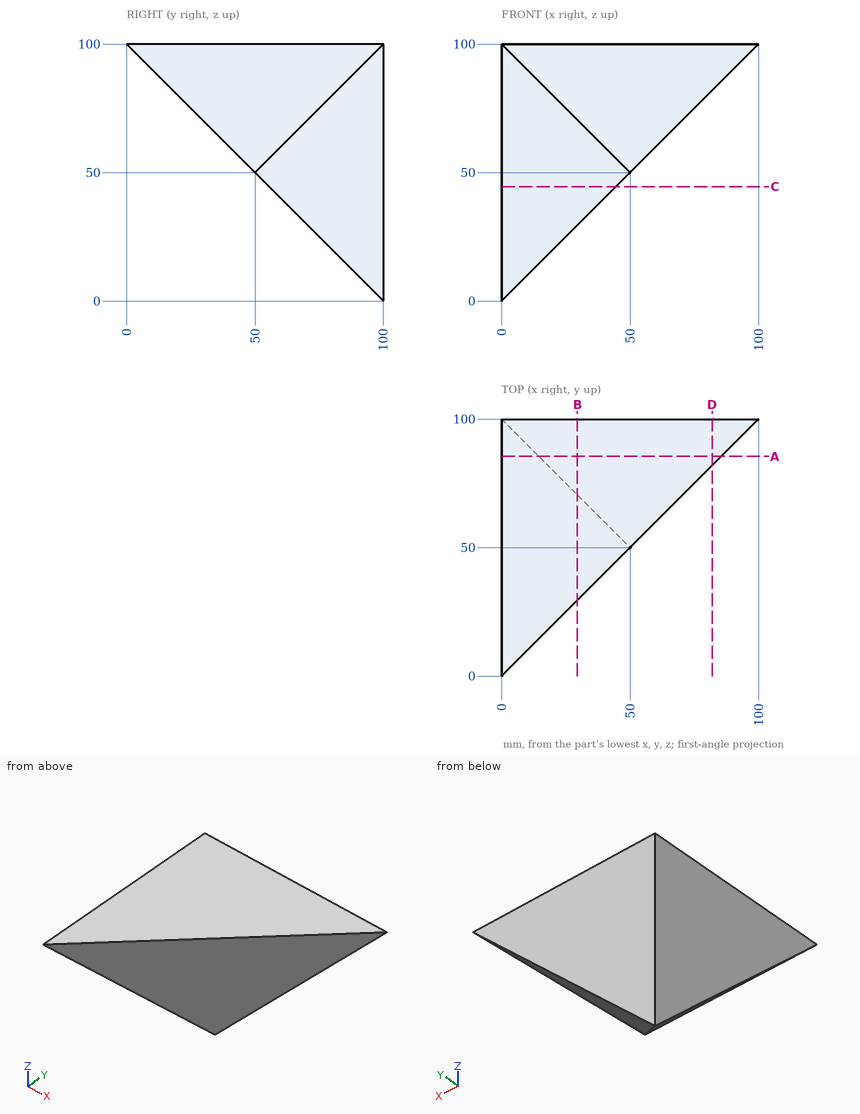
The figure shows three views and two pictorial views of one solid part (mm, origin at its lowest corner). Answer the questions. Round coordinates to 2 decimals unless told otherwise and drop trailing zeros. Order: outer loops, then holes, each group sorted by start corner. A loop starts at its lowest first (then second) coordinate and runs counter-clockwise, first axis right, second up. Notation, with made-up numbers: M 44,37.5 L 100,37.5 A33 cw 100,73.5 Z; hole C 22,62.25 d10. An arc over 180 degrees is marked long. Put each result on its own line as item: value. Start each with the question number.
Q1. Flat-ended cylindrical pins translate along their axes: pin 1 (10 mm diameter, centred on x = 47, y = 69, fed in from -Z); pin 2 (6 mm diameter, centred on x = 28, y = 56.5, fed in from -Z). Find the tip coordinate at first contact, or state that the pin passes through.
Q2. Section C-C, the plane z = 44.5 is taken. Write down the section's boundary in (x, y).
Q3. Section D-D, the plane x = 82 is taken. Write down the section's boundary in (y, z).
Q4. Section A-A, the plane y = 85.5 is taken. Write down the section's boundary in (x, z).
Q5. Section B-B, the plane x = 29.5 is taken. Write down the section's boundary in (y, z), and give its area (3 significant figures).
Q6. Straight lines are drawn through the part: L1, parallel to X at y = 92.5, z = 77; L2, parallel to X at y = 58, z = 89; L3, parallel to Z at x = 35, y = 52.5. For each, find the intervals that lie inside material, in ascending order. Write a range as [from, to].
Findings below:
1. pin 1: stops at z = 42
1. pin 2: stops at z = 40.5
2. outline: M 0,55.5 L 44.5,55.5 L 44.5,100 L 0,100 Z
3. outline: M 82,82 L 100,82 L 100,100 L 82,100 Z
4. outline: M 0,14.5 L 14.5,14.5 L 85.5,85.5 L 85.5,100 L 0,100 Z
5. outline: M 29.5,70.5 L 70.5,29.5 L 100,29.5 L 100,100 L 29.5,100 Z
5. area: 4,130 mm^2
6. L1: x = [0, 77]
6. L2: x = [0, 58]
6. L3: z = [47.5, 100]
